```python
from build123d import *

# Parameters (mm, degrees)
BOSS_EXTRUDE1_DEPTH = 5
SKETCH2_R           = 2.4
CUT_EXTRUDE1_DEPTH  = 3
SKETCH3_R           = 1.25
CUT_EXTRUDE2_DEPTH  = 51.576674466
FILLET1_R           = 2
SKETCH4_R           = 1.75
CUT_EXTRUDE3_DEPTH  = 51.734603576
SKETCH5_R           = 5.315072906
CUT_EXTRUDE4_DEPTH  = 2


with BuildPart() as part:
    # Sketch1 → Boss-Extrude1 (new body)
    with BuildSketch(Plane.XY):
        with BuildLine():
            Line((0, 0), (48, 0))
            ThreePointArc((48, 0), (49.414213562, 0.585786438), (50, 2))
            Line((50, 2), (50, 5))
            ThreePointArc((50, 5), (49.414213562, 6.414213562), (48, 7))
            Line((48, 7), (2, 7))
            ThreePointArc((2, 7), (0.585786438, 6.414213562), (0, 5))
            Line((0, 5), (0, 0))
        make_face()
    extrude(amount=BOSS_EXTRUDE1_DEPTH)

    # Sketch2 → Cut-Extrude1 (cut)
    with BuildSketch(Plane(origin=(0, 0, 0), x_dir=(-1, 0, 0), z_dir=(0, 0, -1))):
        with Locations((-46, 3.5)):
            Circle(SKETCH2_R)
    extrude(amount=-CUT_EXTRUDE1_DEPTH, mode=Mode.SUBTRACT)

    # Sketch3 → Cut-Extrude2 (cut, through all)
    with BuildSketch(Plane(origin=(0, 0, 3), x_dir=(-1, 0, 0), z_dir=(0, 0, -1))):
        with Locations((-46, 3.5)):
            Circle(SKETCH3_R)
    extrude(amount=-CUT_EXTRUDE2_DEPTH, mode=Mode.SUBTRACT)

    # Fillet1
    fillet1_edges = [part.edges().sort_by_distance(p)[0] for p in [
        (49.414213562, 0.585786438, 5),
        (50, 3.5, 5),
        (49.414213562, 6.414213562, 5),
        (25, 7, 5),
        (0.585786438, 6.414213562, 5),
        (0, 2.5, 5),
        (24, 0, 5),
    ]]
    fillet(fillet1_edges, radius=FILLET1_R)

    # Sketch4 → Cut-Extrude3 (cut, through all)
    with BuildSketch(Plane.XY.offset(5)):
        with Locations((4, 3.5)):
            Circle(SKETCH4_R)
    extrude(amount=-CUT_EXTRUDE3_DEPTH, mode=Mode.SUBTRACT)

    # Sketch5 → Cut-Extrude4 (cut)
    with BuildSketch(Plane.XY.offset(5)):
        with Locations((4, 3.5)):
            Circle(SKETCH5_R)
    extrude(amount=-CUT_EXTRUDE4_DEPTH, mode=Mode.SUBTRACT)


solid = part.part
```
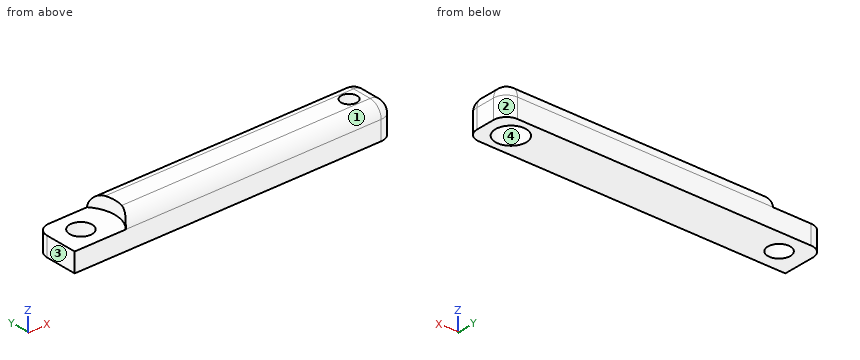
Geometry check sheet. Reference: the model listing, model coordinates, mm. Face numbers are marked on the shaded views. Coordinates: 2 decimals unless noted, no trailing zeros. Order: outer loops, then holes, each group sorted by start corner. A loop starts at its lowest first (then second) coordinate and runs counter-clockwise, first axis right, second up.
Item 1: Section check B-B (x = 4). Enter the section's corners in (y, z).
Item 2: Section check C-C (z = 1.75). Enter the section's corners in (x, y).
Item 3: Section check D-D (z = 3.6). Enter the section's corners in (x, y), plus the area to 3 significant figures.
Item 4: Depth check by flat-ended pin: pin 1 (2 mm diameter, centred on x = 46, y = 3.5, fed in from -Z); pin 2 (2.5 mm diameter, centred on x = 46.5, y = 3.5, fed in from -Z); pin 3 (1 mm diameter, centred on x = 37, y = 5.5, fed in from -Z). Enter the tip coordinate at first touch or a pass-through.
Item 5: Section check A-A (y = 3.5). Enter the section's corners in (x, z).
Item 6: Mould release check, pull along X, two halves, no side actions. Record for the marked faces 1, 2, 3 and 4: released by +X, released by -X, zero draft, split by the parting line, or undercut.
Item 7: Scan lines: line 1 along Y through (x, z) = (46, 1.7); line 2 along Y through (x, z) = (4, 0.75); line 3 along X through (y, z) = (2.75, 0.8). Record each from-to range of solid material in increasing order.
Check sheet entries:
1. outline: (0, 0) - (1.75, 0) - (1.75, 3) - (0, 3) - close; (5.25, 0) - (7, 0) - (7, 3) - (5.25, 3) - close
2. outline: (0, 0) - (48, 0) arc R2 ccw to (50, 2) - (50, 5) arc R2 ccw to (48, 7) - (2, 7) arc R2 ccw to (0, 5) - close; hole circle Ø3.5 at (4, 3.5); hole circle Ø4.8 at (46, 3.5)
3. outline: (8.08, 0.09) - (48, 0.09) arc R1.91 ccw to (49.91, 2) - (49.91, 5) arc R1.91 ccw to (48, 6.91) - (8.08, 6.91) arc R5.32 cw to start; hole circle Ø2.5 at (46, 3.5)
3. area: 273 mm2
4. pin 1: passes through
4. pin 2: stops at z = 3
4. pin 3: stops at z = 0
5. outline: (0, 0) - (2.25, 0) - (2.25, 3) - (0, 3) - close; (5.75, 0) - (43.6, 0) - (43.6, 3) - (44.75, 3) - (44.75, 5) - (9.32, 5) - (9.32, 3) - (5.75, 3) - close; (47.25, 3) - (48.4, 3) - (48.4, 0) - (50, 0) - (50, 3) arc R2 ccw to (48, 5) - (47.25, 5) - close
6. face 1: zero draft
6. face 2: released by +X
6. face 3: released by -X
6. face 4: undercut
7. line 1: y = 0 to 1.1, 5.9 to 7
7. line 2: y = 0 to 1.75, 5.25 to 7
7. line 3: x = 0 to 2.42, 5.58 to 43.72, 48.28 to 50
